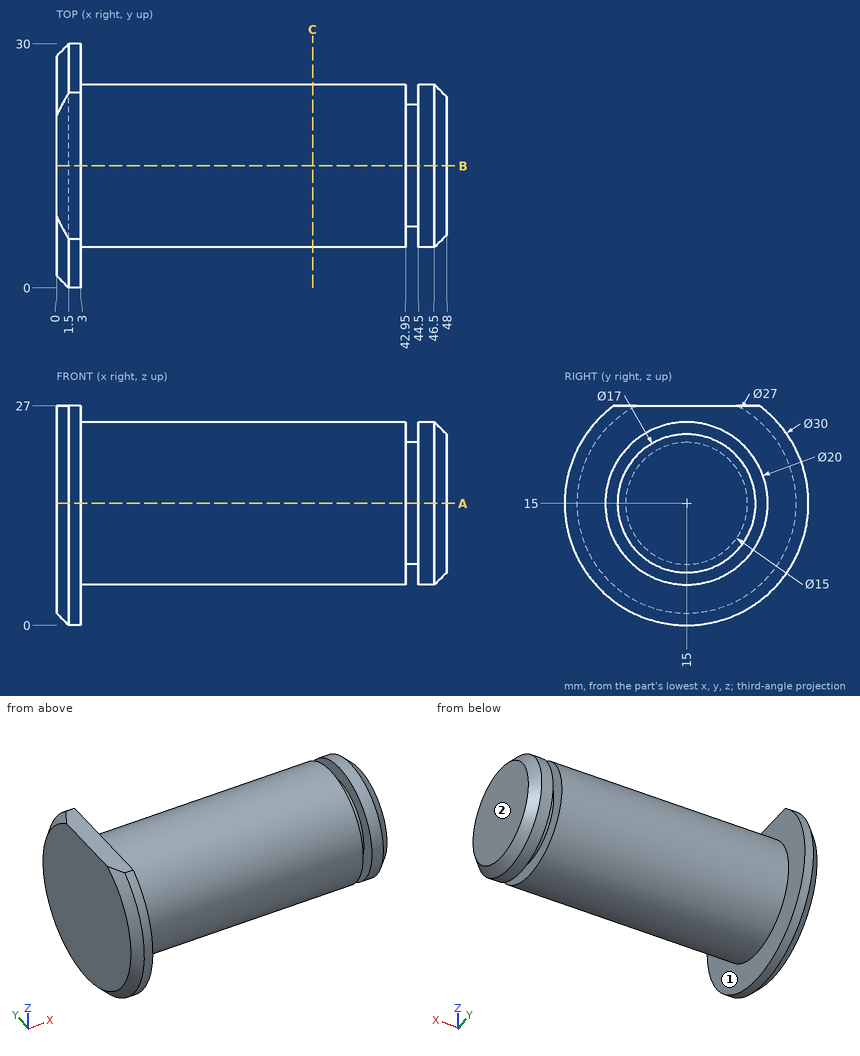
Could you check a few things on this drawing? It's one solid part, dimensions in mm from its lowest x, y, z. A direction names the side the tool comes from. Coordinates: 2 decimals unless noted, no trailing zeros. Order: outer loops, then holes, each group sorted by start corner. A loop starts at its lowest first (then second) coordinate and runs counter-clockwise, first axis right, second up. Notation, with made-up numbers: M 28,-34.75 L 36,-34.75 A13 cw 36,-12.75 Z; hole C -35.5,67 d6. An arc over 180 degrees is marked long. Use one line per item in the form item = value. Start each with the question number.
1. On a 3-axis mill with a long thin cutter (end or side, diameter ignored), from which of +Z, -Z, +X, -X, +Y, -Y can I reach the whole of each face in a straight line? I mean the marked faces 1 and 2. Say none if no direction works.
2. Suppose I cut it at C-C on x = 31.5. Write out the boundary of the cut face in (y, z).
3. Suppose I cut it at B-B on y = 15. Write out the boundary of the cut face in (x, z), then the cut area to 3 significant figures.
4. Suppose I cut it at A-A on z = 15. Write out the boundary of the cut face in (x, y).
5. For pin 1 (1.5 mm diameter, centred on x = 19, z = 15.5, fed in from +Y); pin 2 (4 mm diameter, centred on x = 41.5, y = 19, fed in from +Z); pin 3 (4 mm diameter, centred on y = 4, z = 10.5, fed in from +X), each with a flat end and sliding along its axis, tell me the tip position at first contact or that it passes through.
6. Please list where these lines run through material, in increasing order: line 1 (Y direction, x = 42, z = 14.5); line 2 (Z direction, x = 45, y = 9.75); line 3 (X direction, y = 25.25, z = 9.75).
Geometry says:
q1.face_1 = +X
q1.face_2 = +Z, -Z, +X, +Y, -Y
q2.outline = C 15,15 d20
q3.outline = M 0,1.5 L 1.5,0 L 3,0 L 3,5 L 42.95,5 L 42.95,7.5 L 44.5,7.5 L 44.5,5 L 46.5,5 L 48,6.5 L 48,23.5 L 46.5,25 L 44.5,25 L 44.5,22.5 L 42.95,22.5 L 42.95,25 L 3,25 L 3,27 L 0,27 Z
q3.area = 970 mm^2
q4.outline = M 0,1.5 L 1.5,0 L 3,0 L 3,5 L 42.95,5 L 42.95,7.5 L 44.5,7.5 L 44.5,5 L 46.5,5 L 48,6.5 L 48,23.5 L 46.5,25 L 44.5,25 L 44.5,22.5 L 42.95,22.5 L 42.95,25 L 3,25 L 3,30 L 1.5,30 L 0,28.5 Z
q5.pin_1 = 25
q5.pin_2 = 24.8
q5.pin_3 = 46.62
q6.line_1 = 5.01 to 24.99
q6.line_2 = 6.49 to 23.51
q6.line_3 = 0 to 3
